Verification items for the finished model (mm, model axes). A direction names the side the tool comes from. Coordinates: 2 decimals unless noted, no trailing zeros. Write each loop counter-clockwise with the first axis right and the second up, starting at its lowest first coordinate (ties: lowest second). Pieces come first, ordered by that corner, then holes. Notation, with made-up numbers: (-6.5, -36) - (25.5, -36) arc R24 ccw to (25.5, 3) - close; hole circle Ø4 at (-16, 64.25). An arc over 180 degrees is marked (long way). Use one line per item in the form item = value. Start each with the question number.
(1) Tool access check on faces 4 (the cylindrical face through (-15.567, 3.395, 48.356)), 5 (the flat face through (-3.81, 3, -53)), 6 (the flat face through (1, 50.8, -1)). Record the directions out of +Z, -Z, +X, -X, +Y, -Y that give a thin tool (end or side, any length) a straight path to the whole face; none if there is none.
(2) Gauge pin test, flat ends, axial feed: pin 1 Ø5.5 at (x, y) = (54, 6.5) entering from +Z; pin 2 Ø5.5 at (y, z) = (6.5, 54) entering from +X; pin 3 Ø2.5 at (x, y) = (-53, 3) entering from -Z; pin 4 Ø10 at (x, z) = (36.5, 33) entering from -Y. Record the tip position at first contact, or that the pin passes through.
(3) Mould release check, pull along Y, two halves, no side actions. Record for faces 1 (the flat face through (-46.3, 0, -21.4)), 2 (the cylindrical face through (2.513, 25.044, -57.095)), 3 (the flat face through (-35.4, 5.08, -37.4)): released by +Y, released by -Y, zero draft, split by the parting line, or undercut.
(4) Sectioned sample at D-D (z = 26). Record the cut outline in (x, y), and give its area (3 significant figures).
(5) Sectioned sample at C-C (y = 45.5). Record the cut outline in (x, z), and give its area (3 significant figures).
(6) Sectioned sample at A-A (z = 0). Record the cut outline in (x, y), and give its area (3 significant figures).
(7) Sectioned sample at B-B (x = 0). Record the cut outline in (y, z) (3 decimals), and give its area (3 significant figures).
(8) Material ranges on line 1 (Y direction, x = -12.5, z = -27); line 2 (Z direction, x = 42, y = 5); line 3 (X direction, y = 6, z = -45), recorded low to high. Write a range as [from, to].
from build123d import *
from build123d.topology import SkipClean

# Parameters (mm, degrees)
SKETCH1_R           = 57.15
BOSS_EXTRUDE1_DEPTH = 50.8
CUT_EXTRUDE1_DEPTH  = 8.89
CUT_EXTRUDE3_START  = 6.985
CUT_EXTRUDE3_DEPTH  = 6.985
CUT_EXTRUDE5_START  = 3.81
CUT_EXTRUDE5_DEPTH  = 3.81


with BuildPart() as part:
    # Sketch1 → Boss-Extrude1 (new body)
    with BuildSketch(Plane(origin=(0, 0, 0), x_dir=(1, 0, 0), z_dir=(0, 1, 0))):
        with Locations(Location((0, 0, 0), (0, 0, 270))):
            Circle(SKETCH1_R)
    extrude(amount=BOSS_EXTRUDE1_DEPTH)

    # Sketch2 → Cut-Extrude1 (cut)
    with BuildSketch(Plane.XZ):
        with BuildLine():
            Line((55.749962332, 3.81), (50.656923515, 3.81))
            ThreePointArc((50.656923515, 3.81), (0, 50.8), (-50.656923515, 3.81))
            Line((-50.656923515, 3.81), (-55.749962332, 3.81))
            ThreePointArc((-55.749962332, 3.81), (-55.88, 0), (-55.749962332, -3.81))
            Line((-55.749962332, -3.81), (-50.656923515, -3.81))
            ThreePointArc((-50.656923515, -3.81), (0, -50.8), (50.656923515, -3.81))
            Line((50.656923515, -3.81), (55.749962332, -3.81))
            ThreePointArc((55.749962332, -3.81), (55.88, 0), (55.749962332, 3.81))
        make_face()
    extrude(amount=-CUT_EXTRUDE1_DEPTH, mode=Mode.SUBTRACT)

    # Sketch3 → Cut-Extrude3 (cut)
    with BuildSketch(Plane.XZ.offset(-8.89).offset(CUT_EXTRUDE3_START)):
        with BuildLine():
            Line((3.81, -55.749962332), (3.81, -50.656923515))
            ThreePointArc((3.81, -50.656923515), (0, -50.8), (-3.81, -50.656923515))
            Line((-3.81, -50.656923515), (-3.81, -55.749962332))
            ThreePointArc((-3.81, -55.749962332), (0, -55.88), (3.81, -55.749962332))
        make_face()
        with BuildLine():
            Line((-3.81, 55.749962332), (-3.81, 50.656923515))
            ThreePointArc((-3.81, 50.656923515), (0, 50.8), (3.81, 50.656923515))
            Line((3.81, 50.656923515), (3.81, 55.749962332))
            ThreePointArc((3.81, 55.749962332), (0, 55.88), (-3.81, 55.749962332))
        make_face()
    extrude(amount=-CUT_EXTRUDE3_DEPTH, mode=Mode.SUBTRACT)

    # Sketch4 → Cut-Extrude5 (cut)
    with SkipClean():  # the faces are left unmerged after this step: merging them gives an invalid solid
        with BuildSketch(Plane.XZ.offset(-8.89).offset(CUT_EXTRUDE5_START)):
            with BuildLine():
                Line((55.749962332, 3.81), (50.656923515, 3.81))
                ThreePointArc((50.656923515, 3.81), (35.921024484, 35.921024484), (3.81, 50.656923515))
                Line((3.81, 50.656923515), (3.81, 55.749962332))
                ThreePointArc((3.81, 55.749962332), (39.513126933, 39.513126933), (55.749962332, 3.81))
            make_face()
            with BuildLine():
                Line((-55.749962332, -3.81), (-50.656923515, -3.81))
                ThreePointArc((-50.656923515, -3.81), (-35.921024484, -35.921024484), (-3.81, -50.656923515))
                Line((-3.81, -50.656923515), (-3.81, -55.749962332))
                ThreePointArc((-3.81, -55.749962332), (-39.513126933, -39.513126933), (-55.749962332, -3.81))
            make_face()
        extrude(amount=-CUT_EXTRUDE5_DEPTH, mode=Mode.SUBTRACT)


solid = part.part
Answers below:
q1.face_4 = -Y
q1.face_5 = none
q1.face_6 = +Z, -Z, +X, -X, +Y
q2.pin_1 = 25.29
q2.pin_2 = 25.29
q2.pin_3 = -24.25
q2.pin_4 = 0
q3.face_1 = released by -Y
q3.face_2 = zero draft
q3.face_3 = undercut
q4.outline = (-50.89, 0) - (-43.64, 0) - (-43.64, 8.89) - (49.46, 8.89) - (49.46, 5.08) - (43.64, 5.08) - (43.64, 0) - (50.89, 0) - (50.89, 50.8) - (-50.89, 50.8) - close
q4.area = 4,370 mm2
q5.outline = circle Ø114.3 at (0, 0)
q5.area = 10,300 mm2
q6.outline = (-57.15, 0) - (-55.88, 0) - (-55.88, 8.89) - (55.88, 8.89) - (55.88, 0) - (57.15, 0) - (57.15, 50.8) - (-57.15, 50.8) - close
q6.area = 4,810 mm2
q7.outline = (0, -57.15) - (50.8, -57.15) - (50.8, 57.15) - (0, 57.15) - (0, 50.8) - (1.905, 50.8) - (1.905, 55.88) - (8.89, 55.88) - (8.89, -55.88) - (1.905, -55.88) - (1.905, -50.8) - (0, -50.8) - close
q7.area = 4,830 mm2
q8.line_1 = [8.89, 50.8]
q8.line_2 = [-38.76, -28.58], [28.58, 38.76]
q8.line_3 = [-35.23, -33.13], [23.57, 35.23]
